```python
from build123d import *

# Parameters (mm, degrees)
CHANFRO1_SIZE         = 0.2
ESBO_O5_R             = 2.627342907
CORTE_EXTRUS_O1_DEPTH = 0.5


with BuildPart() as part:
    # Esboço1 → Revolução1 (revolve)
    with BuildSketch(Plane(origin=(0, 0, 0), x_dir=(1, 0, 0), z_dir=(0, 1, 0))):
        Polygon((0, 0), (33, 0), (33, 2.3), (28, 2.3), (28, 2), (11.029645727, 2), (11.029645727, 1.981975223), (11, 1.981975223), (11, 2), (0, 2), align=None)
    revolve(axis=Axis((0, 0, 0), (-1, 0, 0)))

    # Chanfro1
    chanfro1_edges = [part.edges().sort_by_distance(p)[0] for p in [
        (33, 0, 2.3),
    ]]
    chamfer(chanfro1_edges, length=CHANFRO1_SIZE)

    # Esboço5 → Corte-extrusão1 (cut)
    with BuildSketch(Plane.ZY):
        Circle(ESBO_O5_R)
    extrude(amount=-CORTE_EXTRUS_O1_DEPTH, mode=Mode.SUBTRACT)


solid = part.part
```
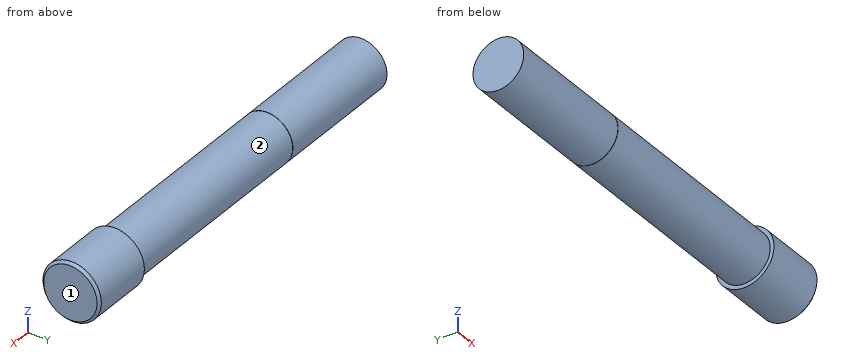
Verification items for the finished model (mm, model axes). Face numbers are marked on the shaded views. A direction names the side the tool comes from. Give positions to 0.01 mm unless a question says otherwise; leave off trailing zeros. Loops run counter-clockwise (first coordinate to the right, second up) from the corner with the lowest first, then second, coordinate; pieces in that order, holes last.
1. Thickness scan on line 1 (X direction, y = 0.75, z = -1.9); line 2 (Z direction, x = 24.5, y = -0.15); line 3 (Z direction, x = 21.5, y = -0.5). Record the ranges inside material, lowest first.
2. Go/stop test with flat-tipped pins: pin 1 Ø1.5 at (x, y) = (10.5, 0) entering from -Z; pin 2 Ø1.5 at (x, z) = (16, -1) entering from -Y; pin 3 Ø1 at (x, y) = (4.5, 1) entering from +Z. Record where each tip stops, or that it passes through.
3. Section check C-C, the plane x = 24. Enter the section's corners in (y, z), then the cut area to 3 significant figures.
4. Set-up check for the marked faces 1 and 2: record each of +Z, -Z, +X, -X, +Y, -Y from which the full face is reachable in a straight line by a thin tool's end or side.
Geometry says:
1. line 1: x = 28 to 33
1. line 2: z = -1.99 to 1.99
1. line 3: z = -1.94 to 1.94
2. pin 1: stops at z = -2
2. pin 2: stops at y = -1.98
2. pin 3: stops at z = 1.94
3. outline: circle Ø4 at (0, 0)
3. area: 12.6 mm2
4. face 1: +Z, -Z, +X, +Y, -Y
4. face 2: -X
